The listing builds one solid part. Answer for the finished solid, in the listing's coordinates (mm). Coordinates: 2 decimals unless noted, no trailing zeros. Loops run counter-clockwise (first coordinate to the right, second up) from the corner with the lowest first, then second, coordinate; pieces in that order, holes last. Notation, with made-up numbers: M 41,-33.5 L 84,-33.5 A27 cw 84,-5.5 Z; hole C 89.25,-35 d1. An arc over 180 degrees is marked long. Return JSON: item names as keys, results as strings. Group by question number.
1. Straight lines are drawn through the part: L1, parallel to Z at x = 1.2, y = 30; L2, parallel to Y at x = 1.2, z = 150; L3, parallel to Z at x = 0.6, y = 52. For each, find the intervals that lie inside material, in ascending order. Write a range as from..to.
2. Section B-B (z = 150) is taken. Write down the section's boundary in (x, y) (3 decimals).
3. Section A-A (y = 10) is taken. Write down the section's boundary in (x, z) (3 decimals), then the cut area to 3 significant figures.
4. Section C-C (x = 2.2) is taken. Count the separate pieces of the cut face and the enclosed holes in it, then the cut area to 3 significant figures.
5. The mould has two halves that part along Y. Classify faces 1 (the face through (1.565, 48.084, 88.243)), 2 (the face through (2, 0, 81)), 3 (the face through (1.61, 59.09, 159.05)): pulls with the +Y half, pulls with the -Y half, needs draft (parallel to the pull), parting line crosses it, or undercut.
Autodesk Inventor part; units mm, degrees
ref_plane "YZ Plane" through (0, 0, 0) normal (1, 0, 0) x (0, 1, 0)
ref_plane "XZ Plane" through (0, 0, 0) normal (0, 1, 0) x (-1, 0, 0)
ref_plane "XY Plane" through (0, 0, 0) normal (0, 0, 1) x (1, 0, 0)
sketch "Sketch1" plane through (0, 0, 0) normal (1, 0, 0) x (0, 1, 0)
  line L0 (0, 0) -> (60, 0)
  line L1 (60, 0) -> (60, 160)
  line L2 (60, 160) -> (0, 160)
  line L3 (0, 160) -> (0, 0)
  line L4 (50, 150) -> (10, 150) construction
  line L5 (10, 150) -> (10, 10) construction
  line L6 (10, 10) -> (50, 10) construction
  line L7 (50, 10) -> (50, 150) construction
  line L8 (50, 80) -> (10, 80) construction
  line L9 (50, 70) -> (10, 70) construction
  line L10 (50, 90) -> (10, 90) construction
  line L11 (30, 150) -> (30, 10) construction
  circle A0 centre (50, 150) radius 2.6
  circle A1 centre (30, 150) radius 2.6
  circle A2 centre (10, 150) radius 2.6
  circle A3 centre (30, 90) radius 2.6
  circle A4 centre (50, 90) radius 2.6
  circle A5 centre (10, 90) radius 2.6
  circle A6 centre (10, 70) radius 2.6
  circle A7 centre (30, 70) radius 2.6
  circle A8 centre (50, 70) radius 2.6
  circle A9 centre (50, 10) radius 2.6
  circle A10 centre (30, 10) radius 2.6
  circle A11 centre (10, 10) radius 2.6
  dimension "d0" = 60
  dimension "d1" = 160
  dimension "d2" = 10
  dimension "d3" = 10
  dimension "d4" = 10
  dimension "d5" = 10
  dimension "d6" = 10
  dimension "d7" = 10
  dimension "d8" = 5.2
  dimension "d9" = 5.2
  dimension "d10" = 5.2
  dimension "d11" = 5.2
  dimension "d12" = 5.2
  dimension "d13" = 5.2
  dimension "d14" = 5.2
  dimension "d15" = 5.2
  dimension "d16" = 5.2
  dimension "d17" = 5.2
  dimension "d18" = 5.2
  dimension "d19" = 5.2
extrude "Extrusion1" add sketch "Sketch1" along normal blind 3.175
fillet "Fillet1" radius 3.175 4 edges at (1.5875, 60, 160) (1.5875, 0, 160) (1.5875, 60, 0) (1.5875, 0, 0)
equation "\"d3\" = d2"
equation "\"d4\" = d2"
equation "\"d5\" = d2"
equation "\"d9\" = d8"
equation "\"d10\" = d8"
equation "\"d11\" = d8"
equation "\"d12\" = d8"
equation "\"d13\" = d8"
equation "\"d14\" = d8"
equation "\"d15\" = d8"
equation "\"d16\" = d8"
equation "\"d17\" = d8"
equation "\"d18\" = d8"
equation "\"d19\" = d8"
properties part number "3x4 2020 Extrusion Gusset Connector"
Worked out:
{
 "1": {"L1": "0..7.4, 12.6..67.4, 72.6..87.4, 92.6..147.4, 152.6..160", "L2": "0..7.4, 12.6..27.4, 32.6..47.4, 52.6..60", "L3": "0..8.34, 11.66..68.34, 71.66..88.34, 91.66..148.34, 151.66..160"},
 "2": {"outline": "M 0,0 L 3.175,0 L 3.175,7.4 L 0,7.4 Z; M 0,12.6 L 3.175,12.6 L 3.175,27.4 L 0,27.4 Z; M 0,32.6 L 3.175,32.6 L 3.175,47.4 L 0,47.4 Z; M 0,52.6 L 3.175,52.6 L 3.175,60 L 0,60 Z"},
 "3": {"outline": "M 0,0 L 3.175,0 L 3.175,7.4 L 0,7.4 Z; M 0,12.6 L 3.175,12.6 L 3.175,67.4 L 0,67.4 Z; M 0,72.6 L 3.175,72.6 L 3.175,87.4 L 0,87.4 Z; M 0,92.6 L 3.175,92.6 L 3.175,147.4 L 0,147.4 Z; M 0,152.6 L 3.175,152.6 L 3.175,160 L 0,160 Z", "area": "442 mm^2"},
 "4": {"separate pieces": "1", "enclosed holes": "12", "area": "9,340 mm^2"},
 "5": {"face 1": "undercut", "face 2": "pulls with the -Y half", "face 3": "pulls with the +Y half"}
}
